CAD build for the part. Positions are in the model's coordinates, mm. A direction names the side the tool comes from. Coordinates: 2 decimals unless noted, no trailing zeros. Loops run counter-clockwise (first coordinate to the right, second up) from the corner with the lowest first, then second, coordinate; pieces in that order, holes last. Notation, with made-up numbers: (75.25, 42) -> (96.25, 42) arc R22 cw to (96.25, 48) -> close; hole circle Ø4 at (83.5, -14.75). An arc over 180 degrees is marked (long way). Write each question's results on one line, items separated by ' | '.
```python
from build123d import *

# Parameters (mm, degrees)
ESBO_O1_W                = 15
ESBO_O1_H                = 26
RESSALTO_EXTRUS_O1_DEPTH = 2.5
RESSALTO_EXTRUS_O2_DEPTH = 4.5
RESSALTO_EXTRUS_O3_DEPTH = 2.15
ESBO_O3_R                = 0.75
CORTE_EXTRUS_O1_DEPTH    = 34.609857185


with BuildPart() as part:
    # Esboço1 → Ressalto-extrusão1 (new body)
    with BuildSketch(Plane.XY):
        with Locations((9, 15)):
            Rectangle(ESBO_O1_W, ESBO_O1_H)
    extrude(amount=RESSALTO_EXTRUS_O1_DEPTH)

    # Esboço1<3> → Ressalto-extrusão2 (add)
    with BuildSketch(Plane.XY):
        Polygon((1.5, 2), (1.5, 28), (0, 28), (0, 0), (18, 0), (18, 28), (16.5, 28), (16.5, 2), align=None)
    extrude(amount=RESSALTO_EXTRUS_O2_DEPTH)

    # Esboço2 → Ressalto-extrusão3 (add)
    with BuildSketch(Plane.XY.offset(2.5)):
        Polygon((1.5, 2), (1.5, 5.5), (2.9, 4.691709623), (2.9, 2.829578102), (4.9, 2.829578102), (4.9, 4.691709623), (5.605720556, 5.5), (6.3, 4.691709623), (6.3, 2.829578102), (8.3, 2.829578102), (8.3, 4.691709623), (9, 5.5), (9.7, 4.691709623), (9.7, 2.829578102), (11.7, 2.829578102), (11.7, 4.691709623), (12.412546272, 5.5), (13.1, 4.691709623), (13.1, 2.829578102), (15.1, 2.829578102), (15.1, 4.691709623), (16.5, 5.5), (16.5, 2), align=None)
    extrude(amount=RESSALTO_EXTRUS_O3_DEPTH)

    # Esboço3 → Corte-extrusão1 (cut, through all)
    with BuildSketch(Plane(origin=(18, 0, 0), x_dir=(0, 0, -1), z_dir=(1, 0, 0))):
        with Locations((-3.5, 3.633303465)):
            Circle(ESBO_O3_R)
    extrude(amount=-CORTE_EXTRUS_O1_DEPTH, mode=Mode.SUBTRACT)


solid = part.part
```
Q1. Drop flat-ended pins along their axis: pin 1 (0.6 mm diameter, centred on x = 10.5, z = 3.5, fed in from +Y); pin 2 (1 mm diameter, centred on x = 9.5, y = 13.5, fed in from +Z); pin 3 (0.6 mm diameter, centred on y = 4, z = 3.5, fed in from +X). Give the stop position or say it passes through.
Results are:
pin 1: y = 2.83 | pin 2: z = 2.5 | pin 3: through
Q2. Cut at A-A on y = 16.5. Write the cut outline in (x, z).
Results are:
outline: (0, 0) -> (18, 0) -> (18, 4.5) -> (16.5, 4.5) -> (16.5, 2.5) -> (1.5, 2.5) -> (1.5, 4.5) -> (0, 4.5) -> close
Q3. Pull direction X, two halves, no side cores. Call faces 3 (the flat face through (11.7, 4.4, 4)), 4 (the flat face through (18, 14, 2)), 5 (the cylindrical face through (12.41, 4.14, 4.053)), 6 (the flat face through (5.95, 5.1, 3.56)): +X half, -X half, draft (parallel to the pull), parting line (faces both ways), or undercut.
Results are:
face 3: undercut | face 4: +X half | face 5: draft | face 6: undercut
Q4. Wall check: L1, parallel to Y at x = 1.25, z = 3.55; L2, parallel to X at y = 19.25, z = 2.55; L3, parallel to Z at x = 14.75, y = 4.25. Give the ranges that are in metal, low to high. Write a range as from..to.
Results are:
L1: 0..2.88, 4.38..28 | L2: 0..1.5, 16.5..18 | L3: 0..2.5
Q5. Cut at C-C on x = 3.75. Write the cut outline in (y, z), and give its area (3 significant figures).
Results are:
outline: (0, 0) -> (28, 0) -> (28, 2.5) -> (2.83, 2.5) -> (2.83, 4.65) -> (2, 4.65) -> (2, 4.5) -> (0, 4.5) -> close | area: 75.8 mm^2
Q6. Cut at B-B on z = 3.5. Give the number of separate pieces and of enclosed holes in the cut face, and give its area (3 significant figures).
Results are:
separate pieces: 6 | enclosed holes: 0 | area: 127 mm^2
Q7. Which spindle directions (+Z, -Z, +X, -X, +Y, -Y) get a long thin tool onto all of the face, cutting with end or side? Do faces 1 (the flat face through (8.3, 4.4, 4)), 2 (the cylindrical face through (9.01, 4.14, 4.053)). Say none if no direction does.
Results are:
face 1: +Z, +Y | face 2: +X, -X
